Could you check a few things on this model? Use its own coordinates, in mm. A direction names the side the tool comes from. Coordinates: 2 decimals unless noted, no trailing zeros. Write each loop counter-clockwise with the first axis right and the second up, starting at its lowest first coordinate (ties: lowest second). Pieces come first, ordered by that corner, then holes.
```python
from build123d import *

# Parameters (mm, degrees)
SKETCH_1_W      = 24.373693789
SKETCH_1_H      = 24.4
EXTRUDE_1_DEPTH = 2
SKETCH_2_W      = 0.399318558
SKETCH_2_H      = 118.043550316
EXTRUDE_2_DEPTH = 132
FILLET_1_R      = 10


with BuildPart() as part:
    # 草图1 → 凸台-拉伸1 (new body)
    with BuildSketch(Plane.XY):
        with Locations((-100.454369689, -61.448491789)):
            Rectangle(SKETCH_1_W, SKETCH_1_H)
    extrude(amount=EXTRUDE_1_DEPTH)

    # 草图2 → 凸台-拉伸2 (add)
    with BuildSketch(Plane.XY.offset(2)):
        with Locations((-88.467182073, -4.716082398)):
            Rectangle(SKETCH_2_W, SKETCH_2_H)
    extrude(amount=EXTRUDE_2_DEPTH)

    # 圆角1
    fillet_1_edges = [part.edges().sort_by_distance(p)[0] for p in [
        (-88.666841352, -56.493174673, 2),
    ]]
    fillet(fillet_1_edges, radius=FILLET_1_R)


solid = part.part
```
1. On a 3-axis mill with a long thin cutter (end or side, diameter ignored), from which of +Z, -Z, +X, -X, +Y, -Y can I reach the whole of each face in a straight line? I mean faces 1 (the face through (-88.5, -63.738, 48.1)), 2 (the face through (-91.518, -56.392, 5.007)), 3 (the face through (-103, -64, 2)). Say none if no direction works.
Verdict:
face 1: +Z, +X, -X, -Y
face 2: +Z, -X, +Y, -Y
face 3: +Z, -X, -Y
2. Please list where these lines run through material, in increasing order: line 1 along X through (y, z) = (-17, 95); line 2 along Z through (x, y) = (-91.5, -54).
Verdict:
line 1: x = -88.67 to -88.27
line 2: z = 0 to 5.03
3. I want a section at A-A on y = -57. Please give me the cut outline in (x, z).
Verdict:
outline: (-112.64, 0) - (-88.27, 0) - (-88.27, 134) - (-88.67, 134) - (-88.67, 12) arc R10 cw to (-98.67, 2) - (-112.64, 2) - close
4. I want a section at C-C on z = 71.5. Please give me the cut outline in (x, y).
Verdict:
outline: (-88.67, -63.74) - (-88.27, -63.74) - (-88.27, 54.31) - (-88.67, 54.31) - close
5. For pin 1 (12 mm diameter, centred on x = -98, y = -53, fed in from +Z); pin 2 (11.5 mm diameter, centred on x = -91.5, z = 66, fed in from -Y), each with a flat end and sliding along its axis, tell me the tip position at first contact or that it passes through.
Verdict:
pin 1: stops at z = 4.55
pin 2: stops at y = -63.74
6. I want a section at B-B on x = -100.25. Please give me the cut outline in (y, z).
Verdict:
outline: (-73.65, 0) - (-49.25, 0) - (-49.25, 2) - (-73.65, 2) - close
